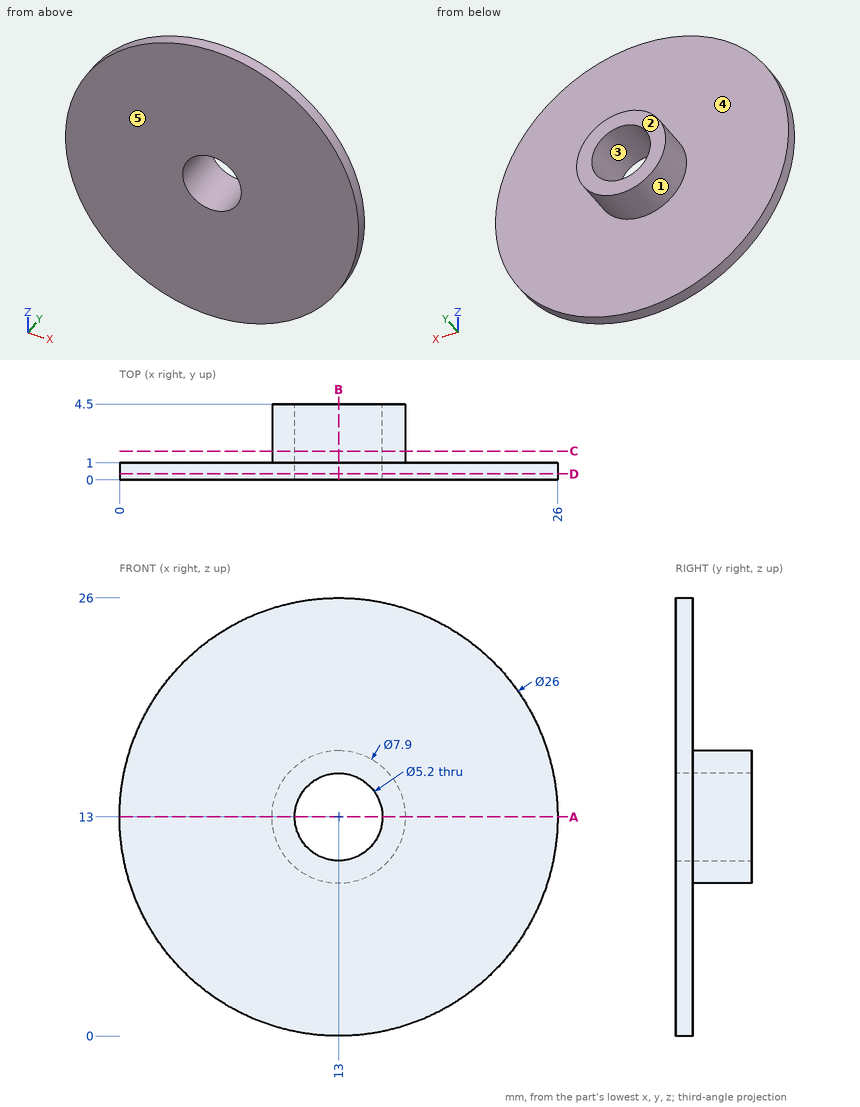
Part print with two shaded views. Sizes in mm from the minimum x, y, z corner. A direction names the side the tool comes from. Round coordinates to 2 decimals unless told otherwise and drop trailing zeros. Order: outer loops, then holes, each group sorted by start corner. A loop starts at its lowest first (then second) coordinate and runs counter-clockwise, first axis right, second up. Notation, with made-up numbers: (31.5, 74) - (88.5, 74) arc R30 ccw to (88.5, 110) - close; hole circle Ø3 at (43.5, 20.5). An arc over 180 degrees is marked (long way). Answer in a Markdown table with one row per item. Add a question column.
(1) Band-saw the part on A-A on z = 13. List the corners of the cut face in (x, y).
(2) Drop flat-ended pins along their axis: pin 1 Ø1.5 at (x, z) = (8, 11) entering from -Y; pin 2 Ø2 at (y, z) = (4, 14.5) entering from +X. Give the stop position or say it passes through.
(3) Mould opens along X. For the marked faces 1, 2 and 3 say: +X half, -X half, draft (parallel to the pull), parting line (faces both ways), or undercut.
(4) 3-axis set-ups, long thin cutter, end or side, ignore diameter. For the marked faces 4 and 5: which of +Z, -Z, +X, -X, +Y, -Y reach the whole face in a straight line?
(5) Band-saw the part on D-D on y = 0.35. List the corners of the cut face in (x, z), and give its area (3 significant figures).
(6) Probe L1, parallel to X at y = 3.2, z = 13; L2, parallel to Y at x = 21.25, z = 23; L3, parallel to Z at x = 11.75, y = 1.05. List the from-to ranges inside material, lowest first. Write a range as [from, to].
(7) Band-saw the part on C-C on y = 1.7. List the corners of the cut face in (x, z).
(8) Band-saw the part on B-B on x = 13. List the corners of the cut face in (y, z), and give its area (4 significant figures).
Data:
| question | item | result |
|---|---|---|
| 1 | outline | (0, 0) - (10.4, 0) - (10.4, 4.5) - (9.05, 4.5) - (9.05, 1) - (0, 1) - close; (15.6, 0) - (26, 0) - (26, 1) - (16.95, 1) - (16.95, 4.5) - (15.6, 4.5) - close |
| 2 | pin 1 | stops at y = 0 |
| 2 | pin 2 | stops at x = 16.92 |
| 3 | face 1 | parting line |
| 3 | face 2 | draft |
| 3 | face 3 | undercut |
| 4 | face 4 | +Y |
| 4 | face 5 | +Z, -Z, +X, -X, -Y |
| 5 | outline | circle Ø26 at (13, 13); hole circle Ø5.2 at (13, 13) |
| 5 | area | 510 mm^2 |
| 6 | L1 | x = [9.05, 10.4], [15.6, 16.95] |
| 6 | L2 | y = [0, 1] |
| 6 | L3 | z = [9.25, 10.72], [15.28, 16.75] |
| 7 | outline | circle Ø7.9 at (13, 13); hole circle Ø5.2 at (13, 13) |
| 8 | outline | (0, 0) - (1, 0) - (1, 9.05) - (4.5, 9.05) - (4.5, 10.4) - (0, 10.4) - close; (0, 15.6) - (4.5, 15.6) - (4.5, 16.95) - (1, 16.95) - (1, 26) - (0, 26) - close |
| 8 | area | 30.25 mm^2 |
